```python
from build123d import *

# Parameters (mm, degrees)
BOSS_EXTRUDE1_DEPTH = 14.5
BOSS_EXTRUDE2_DEPTH = 2
SKETCH9_W           = 1
SKETCH9_H           = 24.94924747
CUT_EXTRUDE7_DEPTH  = 11
SKETCH15_W          = 2
SKETCH15_H          = 25
BOSS_EXTRUDE5_DEPTH = 3.96257304
SKETCH16_W          = 5
SKETCH16_H          = 18
CUT_EXTRUDE8_DEPTH  = 2
FILLET2_R           = 2
SKETCH17_W          = 1
SKETCH17_H          = 20
BOSS_EXTRUDE6_DEPTH = 7


with BuildPart() as part:
    # Sketch1 → Boss-Extrude1 (new, symmetric)
    with BuildSketch(Plane(origin=(0, 0, 0), x_dir=(1, 0, 0), z_dir=(0, 1, 0))):
        Polygon((-43.75, 5.5), (-43.75, -5.5), (43.75, -5.5), (43.75, 5.5), (38.75, 5.5), (38.75, 3.5), (38.75, -3.5), (-38.75, -3.5), (-38.75, 3.5), (-38.75, 5.5), align=None)
    extrude(amount=BOSS_EXTRUDE1_DEPTH, both=True)

    # Sketch8 → Boss-Extrude2 (add)
    with BuildSketch(Plane.XZ.offset(14.5)):
        Polygon((-43.75, 1), (-43.75, -5.5), (-23.804915393, -5.5), (-17.812461495, -5.5), (2.574976796, -9.46257304), (43.75, -9.46257304), (43.75, -8.5), (43.75, -4.5), (43.75, -3), (43.75, -0.96257304), (43.75, 5.5), (-43.75, 5.5), (-43.75, 3), align=None)
    boss_extrude2 = extrude(amount=-BOSS_EXTRUDE2_DEPTH)

    # Mirror1: Boss-Extrude2 across plane
    add(boss_extrude2.mirror(Plane.ZX))

    # Sketch9 → Cut-Extrude7 (cut)
    with BuildSketch(Plane(origin=(0, 0, -5.5), x_dir=(-1, 0, 0), z_dir=(0, 0, -1))):
        with Locations((-41.25, 0.025376265)):
            Rectangle(SKETCH9_W, SKETCH9_H)
        with Locations((41.25, 0.025376265)):
            Rectangle(SKETCH9_W, SKETCH9_H)
    extrude(amount=-CUT_EXTRUDE7_DEPTH, mode=Mode.SUBTRACT)

    # Sketch15 → Boss-Extrude5 (add)
    with BuildSketch(Plane(origin=(0, 0, -5.5), x_dir=(-1, 0, 0), z_dir=(0, 0, -1))):
        with Locations((-42.75, 0)):
            Rectangle(SKETCH15_W, SKETCH15_H)
        with Locations((-39.75, 0)):
            Rectangle(SKETCH15_W, SKETCH15_H)
    extrude(amount=BOSS_EXTRUDE5_DEPTH)

    # Sketch16 → Cut-Extrude8 (cut)
    with BuildSketch(Plane.ZY.offset(-38.75)):
        with Locations((-6.96257304, 0)):
            Rectangle(SKETCH16_W, SKETCH16_H)
    extrude(amount=-CUT_EXTRUDE8_DEPTH, mode=Mode.SUBTRACT)

    # Fillet2
    fillet2_edges = [part.edges().sort_by_distance(p)[0] for p in [
        (43.75, -14.5, -1.98128652),
        (0, -14.5, 5.5),
        (-43.75, -14.5, 0),
        (43.75, 0, 5.5),
        (-43.75, 0, 5.5),
        (-43.75, 14.5, 0),
        (0, 14.5, 5.5),
        (43.75, 14.5, -1.98128652),
    ]]
    fillet(fillet2_edges, radius=FILLET2_R - 0.0001)  # a hair under: the kernel refuses the full size

    # Sketch17 → Boss-Extrude6 (add)
    with BuildSketch(Plane(origin=(0, 0, 3.5), x_dir=(-1, 0, 0), z_dir=(0, 0, -1))):
        with Locations((-13.25, -2.5)):
            Rectangle(SKETCH17_W, SKETCH17_H)
        with Locations((13.25, -2.5)):
            Rectangle(SKETCH17_W, SKETCH17_H)
    extrude(amount=BOSS_EXTRUDE6_DEPTH)


solid = part.part
```
Verification items for the finished model (mm, model axes). A direction names the side the tool comes from. Give positions to 0.01 mm unless a question says otherwise; leave off trailing zeros. Loops run counter-clockwise (first coordinate to the right, second up) from the corner with the lowest first, then second, coordinate; pieces in that order, holes last.
1. Section check B-B, the plane z = -0.75. Enter the section's corners in (x, y), then the cut area to 3 significant figures.
2. Thickness scan on line 1 (X direction, y = 2.25, z = -3); line 2 (Y direction, x = 10, z = -6.25); line 3 (Y direction, x = 13.5, z = 1.5). Record the ranges inside material, lowest first.
3. Set-up check for faces 5 (the flat face through (-40.75, 0, 0)), 6 (the flat face through (-38.75, 0, -1)), 7 (the cylindrical face through (43.18, 13.9, -3.07)): record each of +Z, -Z, +X, -X, +Y, -Y from which the full face is reachable in a straight line by a thin tool's end or side.
4. Go/stop test with flat-tipped pins: pin 1 Ø7.5 at (x, y) = (3.5, 3.5) entering from -Z; pin 2 Ø1.1 at (x, y) = (13.5, -3) entering from -Z. Record where each tip stops, or that it passes through.
5. Section check A-A, the plane y = 9.75. Count the separate pieces of the cut face and the enclosed holes in it, then the cut area to 3 significant figures.
6. Section check C-C, the plane x = -20. Enter the section's corners in (y, z).
7. Mould release check, pull along Y, two halves, no side actions. Record for faces 1 (the flat face through (13.75, -3, 0)), 2 (the flat face through (-7.761, -13.514, -7.454)), 3 (the flat face through (-12.75, -3, 0)), 4 (the cylindrical face through (-43.15, -13.93, -0.94)): released by +Y, released by -Y, zero draft, split by the parting line, or undercut.
Geometry says:
1. outline: (-43.75, -12.5) arc R2 ccw to (-41.75, -14.5) - (41.75, -14.5) arc R2 ccw to (43.75, -12.5) - (43.75, 12.5) arc R2 ccw to (41.75, 14.5) - (-41.75, 14.5) arc R2 ccw to (-43.75, 12.5) - close; hole (-41.75, -12.45) - (-40.75, -12.45) - (-40.75, 12.5) - (-41.75, 12.5) - close; hole (-38.75, -12.5) - (-13.75, -12.5) - (-13.75, 7.5) - (-12.75, 7.5) - (-12.75, -12.5) - (12.75, -12.5) - (12.75, 7.5) - (13.75, 7.5) - (13.75, -12.5) - (38.75, -12.5) - (38.75, 12.5) - (-38.75, 12.5) - close; hole (40.75, -12.45) - (41.75, -12.45) - (41.75, 12.5) - (40.75, 12.5) - close
1. area: 587 mm2
2. line 1: x = -43.75 to -41.75, -40.75 to -38.75, -13.75 to -12.75, 12.75 to 13.75, 38.75 to 40.75, 41.75 to 43.75
2. line 2: y = -14.5 to -12.5, 12.5 to 14.5
2. line 3: y = -14.5 to 7.5, 12.5 to 14.5
3. face 5: +Z, -Z
3. face 6: -Z
3. face 7: +Z, -Z, +X, +Y
4. pin 1: stops at z = 3.5
4. pin 2: stops at z = -3.5
5. separate pieces: 3
5. enclosed holes: 0
5. area: 257 mm2
6. outline: (-14.5, -5.5) - (-12.5, -5.5) - (-12.5, 3.5) - (12.5, 3.5) - (12.5, -5.5) - (14.5, -5.5) - (14.5, 3.5) arc R2 ccw to (12.5, 5.5) - (-12.5, 5.5) arc R2 ccw to (-14.5, 3.5) - close
7. face 1: undercut
7. face 2: zero draft
7. face 3: undercut
7. face 4: released by -Y
